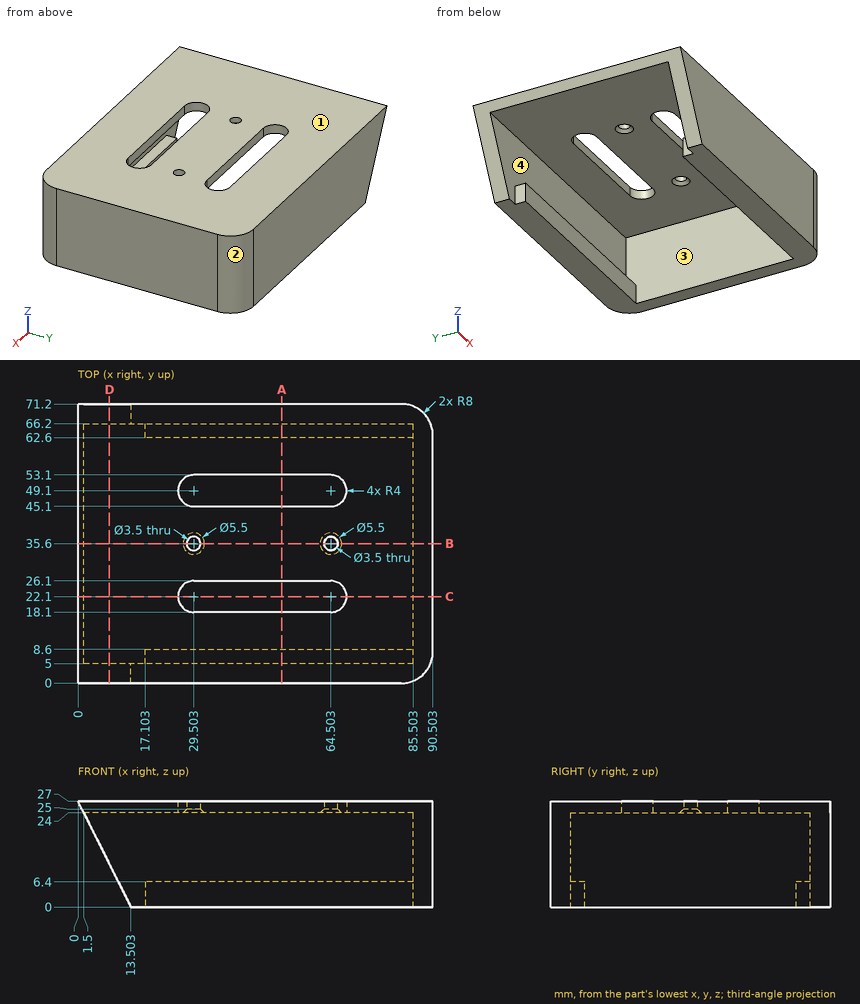
Geometry: see drawing. Coordinates: mm, zero at the bounding-box minimum. Give positions to 0.01 mm unless a question says otherwise; leave off trailing zeros. Write each loop counter-clockwise with the first axis right and the second up, starting at its lowest first coordinate (ties: lowest second). Pieces come first, ordered by that corner, then holes. Notation, with made-up numbers: M 46.25,51 L 65.25,51 A11 cw 65.25,68 Z; hole C 53.25,-38.75 d10. An arc over 180 degrees is marked long. Answer as a JSON object with one key per item and string values.
Q1. Cut plane D-D, the plane x = 8. Return the cut outline in (y, z).
Geometry check:
{"outline": "M 0,11 L 5,11 L 5,24 L 66.2,24 L 66.2,11 L 71.2,11 L 71.2,27 L 0,27 Z"}
Q2. Mould query, pull axis Y, two halves, no side actions, for the marked faces 1, 2, 3 and 4. Classes: +Y half, -Y half, draft (parallel to the pull), parting line (faces both ways), or undercut.
Geometry check:
{"face 1": "draft", "face 2": "+Y half", "face 3": "undercut", "face 4": "undercut"}
Q3. Contact query for flat-ended pins moving along their axis: P1, Ø3, axis at y = 64.5, z = 2.5, coming from the -X side; P2, Ø2, axis at y = 62.5, z = 10.5, coming from the -X side; P3, Ø4.5, axis at x = 29.5, y = 35.6, coming from the -Z side; P4, Ø3, axis at x = 64.5, y = 35.6, coming from the -Z side. Output: stop coordinate, or through.
Geometry check:
{"P1": "stops at x = 17.1", "P2": "stops at x = 85.5", "P3": "stops at z = 24.5", "P4": "passes through"}
Q4. Ray query, line 1 along Y through (x, z) = (50, 8.25); line 2 along Z through (x, y) = (44, 7.5); line 3 along Y through (x, z) = (53.5, 6). Return the intervals inside material, ascending.
Geometry check:
{"line 1": "y = 0 to 5, 66.2 to 71.2", "line 2": "z = 0 to 6.4, 24 to 27", "line 3": "y = 0 to 8.6, 62.6 to 71.2"}
Q5. Cut plane B-B, the plane y = 35.6. Return the cut outline in (x, z), then the cut area to 3 significant figures.
Geometry check:
{"outline": "M 0,27 L 1.5,24 L 26.75,24 L 27.75,25 L 27.75,27 Z; M 31.25,25 L 32.25,24 L 61.75,24 L 62.75,25 L 62.75,27 L 31.25,27 Z; M 66.25,25 L 67.25,24 L 85.5,24 L 85.5,0 L 90.5,0 L 90.5,27 L 66.25,27 Z", "area": "366 mm^2"}
Q6. Cut plane A-A, the plane x = 52. Return the cut outline in (y, z).
Geometry check:
{"outline": "M 0,0 L 8.6,0 L 8.6,6.4 L 5,6.4 L 5,24 L 18.1,24 L 18.1,27 L 0,27 Z; M 26.1,24 L 45.1,24 L 45.1,27 L 26.1,27 Z; M 53.1,24 L 66.2,24 L 66.2,6.4 L 62.6,6.4 L 62.6,0 L 71.2,0 L 71.2,27 L 53.1,27 Z"}
Q7. Cut plane C-C, the plane y = 22.1. Return the cut outline in (x, z).
Geometry check:
{"outline": "M 0,27 L 1.5,24 L 25.5,24 L 25.5,27 Z; M 68.5,24 L 85.5,24 L 85.5,0 L 90.5,0 L 90.5,27 L 68.5,27 Z"}
